Geometry check sheet. Reference: the model listing, model coordinates, mm. A direction names the side the tool comes from. Give positions to 0.01 mm unless a question says otherwise; leave off trailing zeros. Order: outer loops, then holes, each group sorted by start corner. A loop starts at its lowest first (then second) coordinate and runs counter-clockwise, first axis right, second up. Notation, with made-up numbers: M 0.25,69.5 L 35.25,69.5 A27 cw 35.25,108.5 Z; hole C 25.25,62 d6. An arc over 180 degrees is marked long. One line per question, with ' | ' between items. Start each with the question number.
from build123d import *

# Parameters (mm, degrees)
F0_R           = 1.8985
F1_DEPTH       = 3.5
F2_R           = 3
F0_W           = 22
F0_H           = 19
F0_R_2         = 1.75
F3_DEPTH       = 3.5
F4_D           = 3.7973
F4_DEPTH       = 14.38125
F4_CSINK_D     = 7.7978
F4_CSINK_ANGLE = 82
F4_TIP         = 1.1408240143
F5_R           = 3


# Not quite as in the source:
# - a feature names something its author has since deleted; it is built from what else it names


with BuildPart() as f1:
    # F0 (on Top) → F1 (new body)
    with BuildSketch(Plane.XY):
        with BuildLine():
            Line((-32.25, 59.5), (-37.25, 59.5))
            Line((-37.25, 59.5), (-37.25, 54.5))
            ThreePointArc((-37.25, 54.5), (-35.7855339059, 58.0355339059), (-32.25, 59.5))
        make_face()
        with BuildLine():
            Line((37.25, 59.5), (32.25, 59.5))
            ThreePointArc((32.25, 59.5), (35.7855339059, 58.0355339059), (37.25, 54.5))
            Line((37.25, 54.5), (37.25, 59.5))
        make_face()
        with BuildLine():
            ThreePointArc((-32.25, -59.5), (-35.7855339059, -58.0355339059), (-37.25, -54.5))
            Line((-37.25, -54.5), (-37.25, -59.5))
            Line((-37.25, -59.5), (-32.25, -59.5))
        make_face()
        with BuildLine():
            Line((37.25, -59.5), (37.25, -54.5))
            ThreePointArc((37.25, -54.5), (35.7855339059, -58.0355339059), (32.25, -59.5))
            Line((32.25, -59.5), (37.25, -59.5))
        make_face()
        with BuildLine():
            Line((32.25, 59.5), (-32.25, 59.5))
            ThreePointArc((-32.25, 59.5), (-29.5113872125, 58.6833001327), (-27.667424305, 56.5))
            Line((-27.667424305, 56.5), (-11, 56.5))
            Line((-11, 56.5), (11, 56.5))
            Line((11, 56.5), (27.667424305, 56.5))
            ThreePointArc((27.667424305, 56.5), (29.5113872125, 58.6833001327), (32.25, 59.5))
        make_face()
        with BuildLine():
            ThreePointArc((-27.667424305, -56.5), (-29.5113872125, -58.6833001327), (-32.25, -59.5))
            Line((-32.25, -59.5), (32.25, -59.5))
            ThreePointArc((32.25, -59.5), (29.5113872125, -58.6833001327), (27.667424305, -56.5))
            Line((27.667424305, -56.5), (11, -56.5))
            Line((11, -56.5), (-11, -56.5))
            Line((-11, -56.5), (-27.667424305, -56.5))
        make_face()
        with BuildLine():
            ThreePointArc((-34.25, 49.917424305), (-36.4333001327, 51.7613872125), (-37.25, 54.5))
            Line((-37.25, 54.5), (-37.25, -54.5))
            ThreePointArc((-37.25, -54.5), (-36.4333001327, -51.7613872125), (-34.25, -49.917424305))
            Line((-34.25, -49.917424305), (-34.25, 49.917424305))
        make_face()
        with BuildLine():
            Line((37.25, -54.5), (37.25, 54.5))
            ThreePointArc((37.25, 54.5), (36.4333001327, 51.7613872125), (34.25, 49.917424305))
            Line((34.25, 49.917424305), (34.25, -49.917424305))
            ThreePointArc((34.25, -49.917424305), (36.4333001327, -51.7613872125), (37.25, -54.5))
        make_face()
        with BuildLine():
            ThreePointArc((-27.667424305, 56.5), (-29.5113872125, 58.6833001327), (-32.25, 59.5))
            ThreePointArc((-32.25, 59.5), (-35.7855339059, 58.0355339059), (-37.25, 54.5))
            ThreePointArc((-37.25, 54.5), (-36.4333001327, 51.7613872125), (-34.25, 49.917424305))
            Line((-34.25, 49.917424305), (-34.25, 56.5))
            Line((-34.25, 56.5), (-27.667424305, 56.5))
        make_face()
        with BuildLine():
            ThreePointArc((32.25, -59.5), (35.7855339059, -58.0355339059), (37.25, -54.5))
            ThreePointArc((37.25, -54.5), (36.4333001327, -51.7613872125), (34.25, -49.917424305))
            Line((34.25, -49.917424305), (34.25, -56.5))
            Line((34.25, -56.5), (27.667424305, -56.5))
            ThreePointArc((27.667424305, -56.5), (29.5113872125, -58.6833001327), (32.25, -59.5))
        make_face()
        with BuildLine():
            ThreePointArc((-27.25, 54.5), (-27.3554684353, 55.5215482184), (-27.667424305, 56.5))
            Line((-27.667424305, 56.5), (-34.25, 56.5))
            Line((-34.25, 56.5), (-34.25, 49.917424305))
            ThreePointArc((-34.25, 49.917424305), (-29.5113872125, 50.3166998673), (-27.25, 54.5))
        make_face()
        with Locations((-32.25, 54.5)):
            Circle(F0_R, mode=Mode.SUBTRACT)
        with BuildLine():
            ThreePointArc((-27.25, -54.5), (-29.5113872125, -50.3166998673), (-34.25, -49.917424305))
            Line((-34.25, -49.917424305), (-34.25, -56.5))
            Line((-34.25, -56.5), (-27.667424305, -56.5))
            ThreePointArc((-27.667424305, -56.5), (-27.3554684353, -55.5215482184), (-27.25, -54.5))
        make_face()
        with Locations((-32.25, -54.5)):
            Circle(F0_R, mode=Mode.SUBTRACT)
        with BuildLine():
            ThreePointArc((-34.25, -49.917424305), (-36.4333001327, -51.7613872125), (-37.25, -54.5))
            ThreePointArc((-37.25, -54.5), (-35.7855339059, -58.0355339059), (-32.25, -59.5))
            ThreePointArc((-32.25, -59.5), (-29.5113872125, -58.6833001327), (-27.667424305, -56.5))
            Line((-27.667424305, -56.5), (-34.25, -56.5))
            Line((-34.25, -56.5), (-34.25, -49.917424305))
        make_face()
        with BuildLine():
            Line((34.25, -56.5), (34.25, -49.917424305))
            ThreePointArc((34.25, -49.917424305), (28.7144660941, -50.9644660941), (27.667424305, -56.5))
            Line((27.667424305, -56.5), (34.25, -56.5))
        make_face()
        with Locations((32.25, -54.5)):
            Circle(F0_R, mode=Mode.SUBTRACT)
        with BuildLine():
            Line((34.25, 56.5), (27.667424305, 56.5))
            ThreePointArc((27.667424305, 56.5), (28.7144660941, 50.9644660941), (34.25, 49.917424305))
            Line((34.25, 49.917424305), (34.25, 56.5))
        make_face()
        with Locations((32.25, 54.5)):
            Circle(F0_R, mode=Mode.SUBTRACT)
        with BuildLine():
            ThreePointArc((37.25, 54.5), (35.7855339059, 58.0355339059), (32.25, 59.5))
            ThreePointArc((32.25, 59.5), (29.5113872125, 58.6833001327), (27.667424305, 56.5))
            Line((27.667424305, 56.5), (34.25, 56.5))
            Line((34.25, 56.5), (34.25, 49.917424305))
            ThreePointArc((34.25, 49.917424305), (36.4333001327, 51.7613872125), (37.25, 54.5))
        make_face()
        with Locations((-32.25, 54.5)):
            Circle(F0_R)
        with Locations((32.25, 54.5)):
            Circle(F0_R)
        with Locations((-32.25, -54.5)):
            Circle(F0_R)
        with Locations((32.25, -54.5)):
            Circle(F0_R)
    extrude(amount=F1_DEPTH)

    # F2
    f2_edges = [f1.edges().sort_by_distance(p)[0] for p in [
        (-37.25, 59.5, 1.75),
        (37.25, 59.5, 1.75),
        (37.25, -59.5, 1.75),
        (-37.25, -59.5, 1.75),
    ]]
    fillet(f2_edges, radius=F2_R)

    # F0 (on Top) → F3 (join)
    with BuildSketch(Plane.XY):
        with Locations((0, 47)):
            Rectangle(F0_W, F0_H)
        with Locations((0, 42.75)):
            Circle(F0_R_2, mode=Mode.SUBTRACT)
        with Locations((0, -47)):
            Rectangle(F0_W, F0_H)
        with Locations((0, -42.75)):
            Circle(F0_R_2, mode=Mode.SUBTRACT)
    extrude(amount=F3_DEPTH)

    # F4
    with Locations(Plane(origin=(0, 0, 0), x_dir=(1, 0, 0), z_dir=(0, 0, -1))):
        with Locations((-32.25, -54.5), (32.25, -54.5), (32.25, 54.5), (-32.25, 54.5)):
            CounterSinkHole(F4_D / 2, F4_CSINK_D / 2, depth=F4_DEPTH, counter_sink_angle=F4_CSINK_ANGLE)
            with Locations((0, 0, -(F4_DEPTH + F4_TIP / 2))):  # 118° drill point
                Cone(0, F4_D / 2, F4_TIP, mode=Mode.SUBTRACT)

    # F5
    f5_edges = [f1.edges().sort_by_distance(p)[0] for p in [
        (-11, 37.5, 1.75),
        (11, 37.5, 1.75),
        (11, -37.5, 1.75),
        (-11, -37.5, 1.75),
    ]]
    fillet(f5_edges, radius=F5_R)


solid = f1.part
Item 1: Set-up check for faces 1 (the flat face through (-34.25, -1, 2)), 2 (the flat face through (37.25, -1, 2)): record each of +Z, -Z, +X, -X, +Y, -Y from which the full face is reachable in a straight line by a thin tool's end or side.
Item 2: Cross-section at B-B, the plane y = 42.75. Record the cut outline in (x, z).
Item 3: Mould release check, pull along X, two halves, no side actions. Record for faces 3 (the flat face through (-36, -4, 0)), 4 (the cylindrical face through (10.14, -38.4, 1.77)), 5 (the cylindrical face through (-36.39, -58.6, 1.77)): released by +X, released by -X, zero draft, split by the parting line, or undercut.
Item 4: Material ranges on line 1 along Y through (x, z) = (0, 2.5); line 2 along Y through (x, z) = (32.25, 2.65); line 3 along X through (y, z) = (-54.5, 3.2), recorded low to high.
Item 5: Cross-section at C-C, the plane x = 20.5. Record the cut outline in (y, z), plus the area to 3 significant figures.
Item 6: Depth check by flat-ended pin: pin 1 (5 mm diameter, centred on x = -32.25, y = -54.5, fed in from -Z); pin 2 (3.5 mm diameter, centred on x = 32.25, y = 54.5, fed in from -Z). Enter the tip coordinate at first touch or a pass-through.
Item 7: Cross-section at D-D, the plane y = -1. Record the cut outline in (x, z).
Item 8: Cross-section at A-A, the plane x = -32.25. Record the cut outline in (y, z), plus the area to 3 significant figures.
Outcome:
1) face 1: +Z, -Z | face 2: +Z, -Z, +X, +Y, -Y
2) outline: M -37.25,0 L -34.25,0 L -34.25,3.5 L -37.25,3.5 Z; M -11,0 L -1.75,0 L -1.75,3.5 L -11,3.5 Z; M 1.75,0 L 11,0 L 11,3.5 L 1.75,3.5 Z; M 34.25,0 L 37.25,0 L 37.25,3.5 L 34.25,3.5 Z
3) face 3: zero draft | face 4: undercut | face 5: released by -X
4) line 1: y = -59.5 to -44.5, -41 to -37.5, 37.5 to 41, 44.5 to 59.5 | line 2: y = -59.5 to -56.4, -52.6 to -49.5, 49.5 to 52.6, 56.4 to 59.5 | line 3: x = -37.25 to -34.15, -30.35 to -27.25, -11 to 11, 27.25 to 30.35, 34.15 to 37.25
5) outline: M -59.5,0 L -56.5,0 L -56.5,3.5 L -59.5,3.5 Z; M 56.5,0 L 59.5,0 L 59.5,3.5 L 56.5,3.5 Z | area: 21.0 mm²
6) pin 1: stops at z = 1.61 | pin 2: passes through
7) outline: M -37.25,0 L -34.25,0 L -34.25,3.5 L -37.25,3.5 Z; M 34.25,0 L 37.25,0 L 37.25,3.5 L 34.25,3.5 Z
8) outline: M -59.5,0 L -58.4,0 L -56.4,2.3 L -56.4,3.5 L -59.5,3.5 Z; M -52.6,2.3 L -50.6,0 L -49.5,0 L -49.5,3.5 L -52.6,3.5 Z; M 49.5,0 L 50.6,0 L 52.6,2.3 L 52.6,3.5 L 49.5,3.5 Z; M 56.4,2.3 L 58.4,0 L 59.5,0 L 59.5,3.5 L 56.4,3.5 Z | area: 34.2 mm²
